For this review, use the dimensioned drawing (mm, ordinates from the lowest corner) and the shaded views. Round coordinates to 2 decimals unless told otherwise and drop trailing zeros. Loops run counter-clockwise (first coordinate to the right, second up) from the corner with the lowest first, then second, coordinate; pieces in that order, holes last. Notation, with made-up numbers: (78.25, 74.25) - (129.25, 74.25) arc R34 cw to (129.25, 113.25) - close; hole circle Ø9 at (41, -36). An arc over 180 degrees is marked (long way). Use one line per item in the form item = value. Start each with the question number.
(1) We need section B-B, the plane z = 61.75. Write out the cut boundary in (x, y).
(2) Wall thickness on probe 1 along X at (y, z) = (1.65, 61.75); probe 2 along X at (y, z) = (1.6, 44); probe 3 along Z at (x, y) = (11, 2.7): over which ranges is each line inside the solid? List them lowest first. Write a range as [from, to].
(3) We need section A-A, the plane x = 7. Write out the cut boundary in (y, z), then the cut area to 3 significant figures.
(4) We need section C-C, the plane x = 69.5. Write out the cut boundary in (y, z).
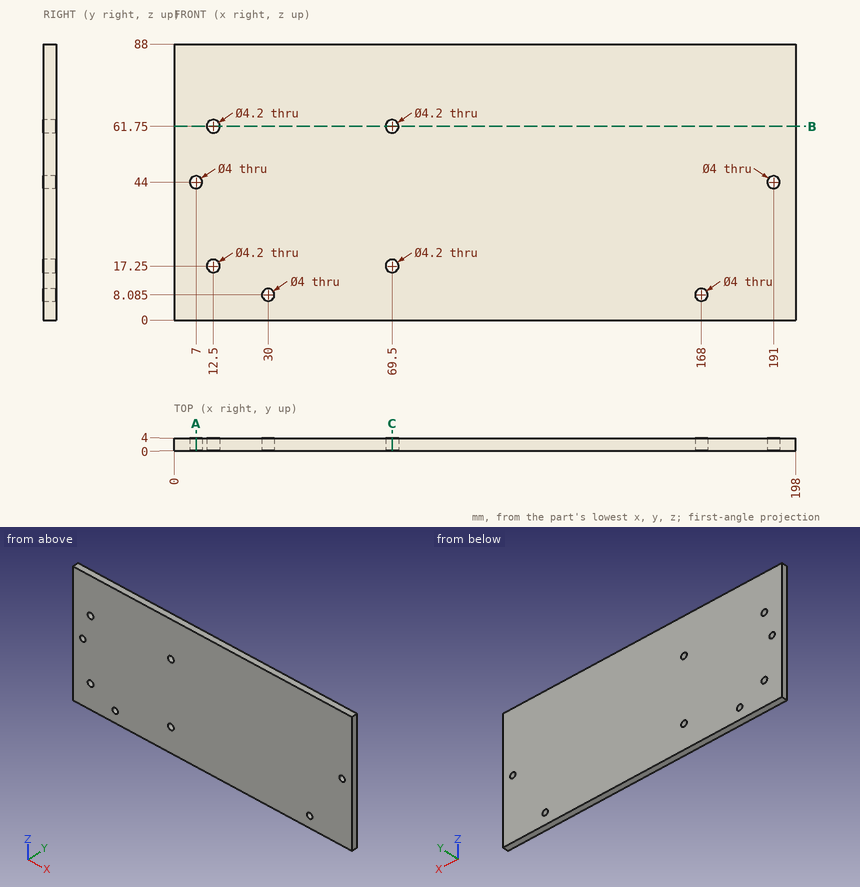
Data:
q1.outline = (0, 0) - (10.4, 0) - (10.4, 4) - (0, 4) - close; (14.6, 0) - (67.4, 0) - (67.4, 4) - (14.6, 4) - close; (71.6, 0) - (198, 0) - (198, 4) - (71.6, 4) - close
q2.probe_1 = [0, 10.4], [14.6, 67.4], [71.6, 198]
q2.probe_2 = [0, 5], [9, 189], [193, 198]
q2.probe_3 = [0, 15.78], [18.72, 60.28], [63.22, 88]
q3.outline = (0, 0) - (4, 0) - (4, 42) - (0, 42) - close; (0, 46) - (4, 46) - (4, 88) - (0, 88) - close
q3.area = 336 mm^2
q4.outline = (0, 0) - (4, 0) - (4, 15.15) - (0, 15.15) - close; (0, 19.35) - (4, 19.35) - (4, 59.65) - (0, 59.65) - close; (0, 63.85) - (4, 63.85) - (4, 88) - (0, 88) - close
